from build123d import *

# Parameters (mm, degrees)
FILLET2_R           = 0.2413
CUT_EXTRUDE2_DEPTH  = 26.574028913
CIRPATTERN1_COUNT   = 16
SKETCH10_R          = 29.093421686
CUT_EXTRUDE3_DEPTH  = 15.24
SKETCH11_R          = 20.555223038
CUT_EXTRUDE4_DEPTH  = 10.16
SKETCH12_R          = 7.917123479
SKETCH12_R_2        = 4.826
BOSS_EXTRUDE1_DEPTH = 6.35
SKETCH_1_R          = 1.4351
CUT_EXTRUDE_1_DEPTH = 24.590352248


with BuildPart() as part:
    # Sketch4 → Revolve1 (revolve)
    with BuildSketch(Plane(origin=(0, 0, 0), x_dir=(0, 0, -1), z_dir=(1, 0, 0))):
        Polygon((-31.75, 6.35), (-31.75, 10.3251), (-19.05, 10.3251), (-19.05, 12.065), (0, 12.065), (0, 6.35), align=None)
    revolve(axis=Axis((0, 0, 19.05), (0, 0, 1)))

    # Fillet2
    fillet2_edges = [part.edges().sort_by_distance(p)[0] for p in [
        (0, -12.065, 0),
        (0, -12.065, 19.05),
        (0, -10.3251, 19.05),
        (0, -10.3251, 31.75),
    ]]
    fillet(fillet2_edges, radius=FILLET2_R)

    # Sketch7 → Cut-Extrude2 (cut, through all)
    with BuildSketch(Plane.XY.offset(19.05)):
        with BuildLine():
            ThreePointArc((-0.107661594, 8.790121954), (0, 8.79078125), (0.107661594, 8.790121954))
            ThreePointArc((0.107661594, 8.790121954), (0.342591452, 8.864525037), (0.487011309, 9.064201678))
            ThreePointArc((0.487011309, 9.064201678), (1.083642605, 10.543346068), (1.897871283, 11.914793728))
            ThreePointArc((1.897871283, 11.914793728), (0, 12.065), (-1.897871283, 11.914793728))
            ThreePointArc((-1.897871283, 11.914793728), (-1.083642605, 10.543346068), (-0.487011309, 9.064201678))
            ThreePointArc((-0.487011309, 9.064201678), (-0.342591452, 8.864525037), (-0.107661594, 8.790121954))
        make_face()
    cut_extrude2 = extrude(amount=-CUT_EXTRUDE2_DEPTH, mode=Mode.SUBTRACT)

    # CirPattern1: Cut-Extrude2 ×16 about axis
    cirpattern1_axis = Axis((0, 0, 0), (0, 0, 1))
    for i in range(1, CIRPATTERN1_COUNT):
        add(cut_extrude2.rotate(cirpattern1_axis, i * 360 / CIRPATTERN1_COUNT), mode=Mode.SUBTRACT)

    # Sketch10 → Cut-Extrude3 (cut)
    with BuildSketch(Plane.XY.offset(31.75)):
        Circle(SKETCH10_R)
    extrude(amount=-CUT_EXTRUDE3_DEPTH, mode=Mode.SUBTRACT)

    # Sketch11 → Cut-Extrude4 (cut)
    with BuildSketch(Plane(origin=(0, 0, 0), x_dir=(-1, 0, 0), z_dir=(0, 0, -1))):
        Circle(SKETCH11_R)
    extrude(amount=-CUT_EXTRUDE4_DEPTH, mode=Mode.SUBTRACT)

    # Sketch12 → Boss-Extrude1 (add)
    with BuildSketch(Plane.XY.offset(16.51)):
        Circle(SKETCH12_R)
        Circle(SKETCH12_R_2, mode=Mode.SUBTRACT)
    extrude(amount=-BOSS_EXTRUDE1_DEPTH)

    # Эскиз1 → Вырез-Вытянуть1 (cut, through all)
    with BuildSketch(Plane(origin=(0, 0, 0), x_dir=(-1, 0, 0), z_dir=(0, 0, -1))):
        with Locations(Location((6.601034981, 4.40797498, 0), (0, 0, 90))):
            Circle(SKETCH_1_R)
        with Locations(Location((4.40797498, -6.601034981, 0), (0, 0, 90))):
            Circle(SKETCH_1_R)
        with Locations(Location((-6.601034981, -4.40797498, 0), (0, 0, 90))):
            Circle(SKETCH_1_R)
        with Locations(Location((-4.40797498, 6.601034981, 0), (0, 0, 90))):
            Circle(SKETCH_1_R)
    extrude(amount=-CUT_EXTRUDE_1_DEPTH, mode=Mode.SUBTRACT)


solid = part.part
The listing builds one solid part. Answer for the finished solid, in the listing's coordinates (mm). A direction names the side the tool comes from. Round coordinates to 2 decimals unless told otherwise and drop trailing zeros. Order: outer loops, then holes, each group sorted by start corner. A loop starts at its lowest first (then second) coordinate and runs counter-clockwise, first axis right, second up. Notation, with made-up numbers: (-5.75, 7) -> (-1.75, 7) arc R36 cw to (-1.75, 45) -> close; hole circle Ø10 at (-21, 59). An arc over 180 degrees is marked (long way). One line per item, written item: value.
Item 1: Find section B-B, the plane x = 1.25. Give the vertices of the cut face in (y, z), then the cut area to 3 significant figures.
Taken from the geometry:
outline: (-10.87, 10.16) -> (-4.66, 10.16) -> (-4.66, 16.51) -> (-10.87, 16.51) -> close; (4.66, 10.16) -> (10.87, 10.16) -> (10.87, 16.51) -> (4.66, 16.51) -> close
area: 78.8 mm2
Item 2: For faces 4 (the cylindrical face through (-10.133, -3.035, 13.379)), 5 (the cylindrical face through (9.34, 5.05, 13.38)), 6 (the cylindrical face through (5.05, -9.34, 13.38)), determine the directions among +Z, -Z, +X, -X, +Y, -Y from which every point of the face is accessible in a straight line to the end or side of a thin tool.
Taken from the geometry:
face 4: +Z, -Z
face 5: +Z, -Z, +X
face 6: +Z, -Z, -Y
Item 3: Given P1, Ø1, axis at x = 7.5, y = -8, coming from the -Z side, flat-ended and moving along its own axis, determine where the tip first touches the part or whether it passes through.
Taken from the geometry:
P1: passes through
Item 4: Find section C-C, the plane z = 10.75. State how many separate pieces and enclosed holes the cut face has, then the cut area to 3 significant figures.
Taken from the geometry:
separate pieces: 1
enclosed holes: 5
area: 248 mm2
Item 5: For a pull along Y with two mould halves and no side action, classify faces 1 (the cylindrical face through (-5.02, -9.31, 13.38)), 2 (the cylindrical face through (11.834, 2.347, 13.291)), 3 (the cylindrical face through (8.024, -4.595, 13.291)) as released by +Y, released by -Y, zero draft, split by the parting line, or undercut.
Taken from the geometry:
face 1: released by -Y
face 2: released by +Y
face 3: undercut
Item 6: Straight lines are drawn through the part: L1, parallel to X at y = 8.5, z = 14.75; L2, parallel to X at y = 4, z = 13; L3, parallel to Y at x = 9.5, z = 15.25. For each, find the intervals that lie inside material, in ascending order.
Taken from the geometry:
L1: x = -6.78 to -4.19, -3.02 to 3.02, 4.19 to 6.78
L2: x = -8.28 to -7.98, -5.23 to -2.7, 2.7 to 8.28
L3: y = -7.03 to -5.24, -3.06 to -0.64, 0.64 to 3.06, 5.24 to 7.03
Item 7: Find section A-A, the plane y = 5.5. Give the vertices of the cut face in (x, z).
Taken from the geometry:
outline: (-9.71, 10.16) -> (-7.53, 10.16) -> (-7.53, 16.51) -> (-9.71, 16.51) -> close; (-5.67, 10.16) -> (3.49, 10.16) -> (3.49, 16.51) -> (-5.67, 16.51) -> close; (5.33, 10.16) -> (9.71, 10.16) -> (9.71, 16.51) -> (5.33, 16.51) -> close
